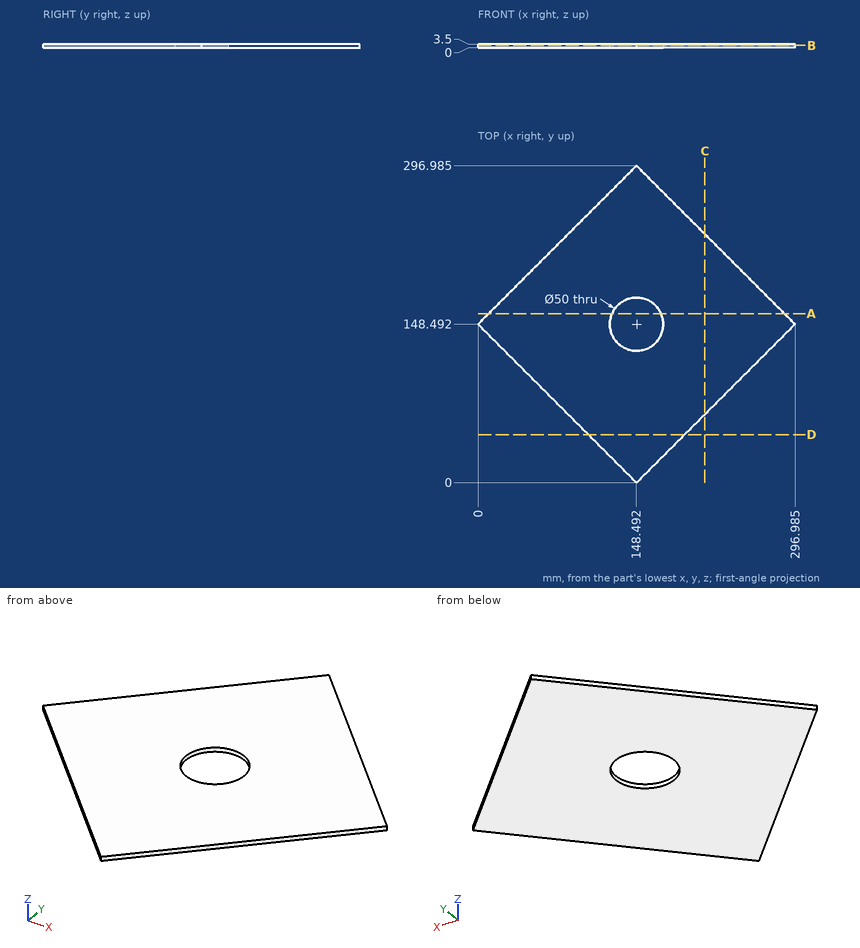
Study the drawing (mm; zero at the part's minimum x, y, z) and answer. Give positions to 0.01 mm unless a question says otherwise; leave off trailing zeros. Write each loop counter-clockwise with the first axis right and the second up, starting at its lowest first coordinate (ties: lowest second). Pieces come first, ordered by that corner, then holes. Notation, with made-up numbers: (-36.75, 88.5) -> (-25.75, 88.5) arc R11 ccw to (-25.75, 107.5) -> close; hole circle Ø3 at (55.25, 53). An arc over 180 degrees is marked (long way). Answer as a JSON object with one key per item and string values. Group by question number.
1) Find section D-D (y = 45). Write down the section's boundary in (x, z), and give its area (3 significant figures).
2) Consider L1, parallel to Y at x = 272, z = 2.7 (1 decimal); L2, parallel to X at y = 138, z = 0.3 (1 decimal); L3, parallel to X at y = 149, z = 0.2 (1 decimal). Determine where each line is inside the solid, lowest interval first. Write a range as from..to.
3) Find section B-B (z = 2.3). Write down the section's boundary in (x, y) (1 decimal), and give its area (3 significant figures).
4) Each of these flat-tipped pins is pushed along its axis until it touches: P1, Ø2, axis at y = 256, z = 2.5, coming from the -X side; P2, Ø1, axis at x = 193.5, z = 1.5, coming from the +Y side; P3, Ø2, axis at y = 175.5, z = 1.5, coming from the -X side. Where does it stop, or does it pass through?
5) Find section C-C (x = 212.5). Write down the section's boundary in (y, z).
6) Find section A-A (y = 158.5). Write down the section's boundary in (x, z).
Values follow:
{
 "1": {"outline": "(103.49, 0) -> (193.49, 0) -> (193.49, 3.5) -> (103.49, 3.5) -> close", "area": "315 mm2"},
 "2": {"L1": "y = 123.5..173.5", "L2": "x = 10.5..125.8, 171.2..286.5", "L3": "x = 0.5..123.5, 173.5..296.5"},
 "3": {"outline": "(0, 148.5) -> (148.5, 0) -> (297, 148.5) -> (148.5, 297) -> close; hole circle Ø50 at (148.5, 148.5)", "area": "42,100 mm2"},
 "4": {"P1": "stops at x = 106.51", "P2": "stops at y = 252.48", "P3": "stops at x = 26.01"},
 "5": {"outline": "(64.01, 0) -> (232.98, 0) -> (232.98, 3.5) -> (64.01, 3.5) -> close"},
 "6": {"outline": "(10.01, 0) -> (125.58, 0) -> (125.58, 3.5) -> (10.01, 3.5) -> close; (171.4, 0) -> (286.98, 0) -> (286.98, 3.5) -> (171.4, 3.5) -> close"}
}
